Autodesk Inventor part; units mm, degrees
ref_plane "YZ Plane" through (0, 0, 0) normal (1, 0, 0) x (0, 1, 0)
ref_plane "XZ Plane" through (0, 0, 0) normal (0, 1, 0) x (-1, 0, 0)
ref_plane "XY Plane" through (0, 0, 0) normal (0, 0, 1) x (1, 0, 0)
sketch "Sketch1" plane through (0, 0, 0) normal (0, 1, 0) x (-1, 0, 0)
  line L0 (2.54, 0) -> (25.4, 0)
  line L1 (0, 25.4) -> (0, 2.54)
  line L2 (22.86, 4.7625) -> (7.3025, 4.7625)
  line L3 (4.7625, 7.3025) -> (4.7625, 22.86)
  line L4 (2.2225, 25.4) -> (0, 25.4)
  line L5 (25.4, 2.2225) -> (25.4, 0)
  arc A0 (4.7625, 7.3025) -> (7.3025, 4.7625) centre (7.3025, 7.3025) ccw
  arc A1 (4.7625, 22.86) -> (2.2225, 25.4) centre (2.2225, 22.86) ccw
  arc A2 (0, 2.54) -> (2.54, 0) centre (2.54, 2.54) ccw
  arc A3 (25.4, 2.2225) -> (22.86, 4.7625) centre (22.86, 2.2225) ccw
  point P0 (0, 0)
  dimension "d2" = 4.7625
  dimension "d3" = 25.4
  dimension "d4" = 25.4
  dimension "d5" = 2.54
extrude "Back Leg" add sketch "Sketch1" along normal blind 1524
properties part number "legs-bl_t"
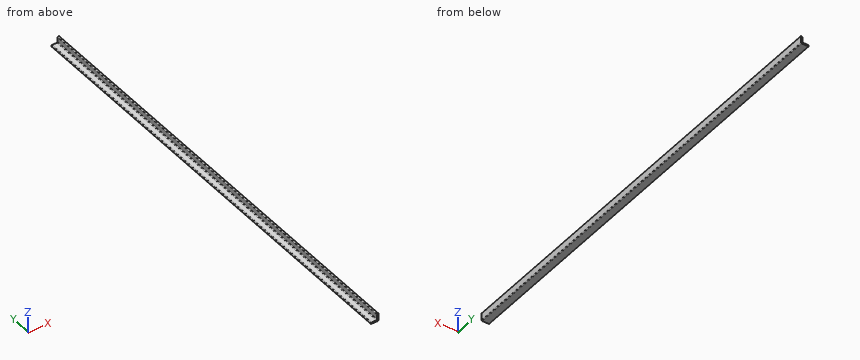
Model file for the job. Use its own axes, mm. Give positions to 0.01 mm unless a question says otherwise; leave off trailing zeros. Write each loop counter-clockwise with the first axis right and the second up, starting at its lowest first coordinate (ties: lowest second). Pieces come first, ordered by that corner, then holes. Notation, with made-up numbers: (-7, 78.25) -> (31, 78.25) arc R22 cw to (31, 86.25) -> close; hole circle Ø4 at (8.5, 16). An arc over 180 degrees is marked (long way). Use CSV: the item, a comma, the result in double quotes. Start each with the question number.
1) Cut at A-A on y = 1051. List the corners of the cut face in (x, z).
2) Cut at B-B on z = 13.25. List the corners of the cut face in (x, y).
3) Pin check, flat tips, straight feed: P1, Ø12.5, axis at y = 491, z = 18.5, coming from the -X side; P2, Ø8, axis at x = -4, y = 496, coming from the -Z side; P3, Ø8, axis at x = -16, z = 10.5, coming from the +Y side; P4, Ø3, axis at x = -13.5, y = 565, coming from the +Z side. Stop position of each tip, or through.
4) Cut at C-C on x = -13.5. List the corners of the cut face in (y, z).
5) Drill centre lines: L1, parallel to X at y = 162.5, z = 7.5; L2, parallel to Z at x = -11.25, y = 816; L3, parallel to X at y = 324, z = 1.75. Where is each one in solid material? Low to high.
Final values:
1,outline,"(-25.4, 0) -> (-2.54, 0) arc R2.54 ccw to (0, 2.54) -> (0, 25.4) -> (-2.22, 25.4) arc R2.54 ccw to (-4.76, 22.86) -> (-4.76, 7.3) arc R2.54 cw to (-7.3, 4.76) -> (-22.86, 4.76) arc R2.54 ccw to (-25.4, 2.22) -> close"
2,outline,"(-4.76, 0) -> (0, 0) -> (0, 1524) -> (-4.76, 1524) -> close"
3,P1,"stops at x = -4.76"
3,P2,"stops at z = 0"
3,P3,"passes through"
3,P4,"stops at z = 4.76"
4,outline,"(0, 0) -> (1524, 0) -> (1524, 4.76) -> (0, 4.76) -> close"
5,L1,"x = -4.76 to 0"
5,L2,"z = 0 to 4.76"
5,L3,"x = -25.4 to -0.13"
